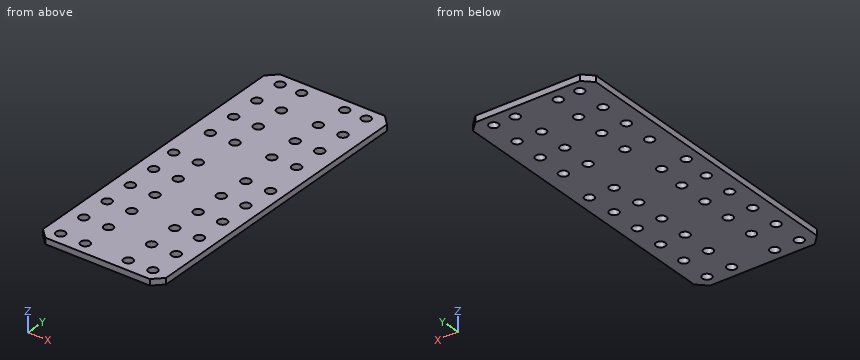
Autodesk Inventor part; units mm, degrees
ref_plane "YZ Plane" through (0, 0, 0) normal (1, 0, 0) x (0, 1, 0)
ref_plane "XZ Plane" through (0, 0, 0) normal (0, 1, 0) x (-1, 0, 0)
ref_plane "XY Plane" through (0, 0, 0) normal (0, 0, 1) x (1, 0, 0)
sketch "Sketch1" plane through (0, 0, 0) normal (0, 0, 1) x (1, 0, 0)
  circle A0 centre (-11, -99.1166) radius 1.5
  circle A1 centre (-13, -89.1166) radius 1.5
  circle A2 centre (-5, -89.1166) radius 1.5
  line L0 (0, -100.499) -> (0, -85.1166)
  line L1 (0, -85.1166) -> (-20, -85.1166)
  line L2 (-20, -85.1166) -> (-20, -111.0877)
  line L3 (-20, -111.0877) -> (-11.9783, -111.0877)
  line L4 (-11.9783, -111.0877) -> (-7.95, -105.7166)
  arc A3 (0, -100.499) -> (-7.95, -105.7166) centre (3.25, -114.1166) ccw
  circle A4 centre (-29, -99.1166) radius 1.5
  circle A5 centre (-27, -89.1166) radius 1.5
  circle A6 centre (-35, -89.1166) radius 1.5
  line L5 (-40, -100.499) -> (-40, -85.1166)
  arc A7 (-32.05, -105.7166) -> (-40, -100.499) centre (-43.25, -114.1166) ccw
  line L6 (-28.0217, -111.0877) -> (-32.05, -105.7166)
  line L7 (-20, -111.0877) -> (-28.0217, -111.0877)
  line L8 (-20, -85.1166) -> (-20, -111.0877)
  line L9 (-40, -85.1166) -> (-20, -85.1166)
  circle A8 centre (-6, 4) radius 1.5
  circle A9 centre (-10, 13) radius 1.5
  circle A10 centre (-13, 4) radius 1.5
  line L10 (-10, 23) -> (-10, 40)
  line L11 (-20, 40) -> (-10, 40)
  line L12 (-20, 0) -> (-20, 40)
  line L13 (0, 0) -> (-20, 0)
  line L14 (0, 0) -> (0, 8)
  line L15 (0, 8) -> (-10, 23)
  circle A11 centre (-34, 4) radius 1.5
  circle A12 centre (-30, 13) radius 1.5
  circle A13 centre (-27, 4) radius 1.5
  line L16 (-30, 23) -> (-30, 40)
  line L17 (-40, 8) -> (-30, 23)
  line L18 (-40, 0) -> (-40, 8)
  line L19 (-40, 0) -> (-20, 0)
  line L20 (-20, 0) -> (-20, 40)
  line L21 (-20, 40) -> (-30, 40)
  line L22 (0, 0) -> (-40, 0)
  line L23 (-40, 0) -> (-40, 8)
  line L24 (-40, 8) -> (0, 8)
  line L25 (0, 8) -> (0, 0)
  line L26 (0, -85.1166) -> (-40, -85.1166)
  line L27 (-40, -85.1166) -> (-40, -93.1166)
  line L28 (-40, -93.1166) -> (0, -93.1166)
  line L29 (0, -93.1166) -> (0, -85.1166)
  line L30 (0, -85.1166) -> (-40, -85.1166)
  line L31 (-40, -85.1166) -> (-40, 0)
  line L32 (-40, 0) -> (0, 0)
  line L33 (0, 0) -> (0, -85.1166)
  point P0 (0, -93.1166)
  dimension "d0" = 40
  dimension "d1" = 8
  dimension "d2" = 40
  dimension "d3" = 8
extrude "Extrusion1" add sketch "Sketch1" along normal blind 2 contours L28 L2 L1 L0 | L1 L9 L31 L19 L13 L33 | L28 L5 L9 L2 | L13 L12 L24 L14 | L19 L18 L24 L12
sketch "Sketch2" plane through (0, 0, 0) normal (0, 0, -1) x (-1, 0, 0)
  circle A0 centre (12.2614, -39.5) radius 1.5
  circle A1 centre (4.2614, -39.5) radius 1.5
  point P0 (0, 0)
extrude "Extrusion2" cut sketch "Sketch2" against normal blind 10
ref_plane "Work Plane1" through (-20, -93.1166, 0) normal (1, 0, 0) x (0, 0, -1)
mirror "Mirror1" about plane through (-20, -93.1166, 0) normal (1, 0, 0) of "Extrusion2"
sketch "Sketch3" plane through (0, 0, 0) normal (0, 0, -1) x (-1, 0, 0)
  circle A0 centre (35.7386, -39.5) radius 1.5
  circle A1 centre (27.7386, -39.5) radius 1.5
  circle A2 centre (4.2614, -39.5) radius 1.5
  circle A3 centre (12.2614, -39.5) radius 1.5
  line L0 (40, 8) -> (40, -93.1166)
  line L1 (0, 8) -> (40, 8)
  line L2 (0, -93.1166) -> (0, 8)
  line L3 (40, -93.1166) -> (0, -93.1166)
  circle A4 centre (13, 4) radius 1.5
  circle A5 centre (6, 4) radius 1.5
  circle A6 centre (27, 4) radius 1.5
  circle A7 centre (34, 4) radius 1.5
  circle A8 centre (35, -89.1166) radius 1.5
  circle A9 centre (27, -89.1166) radius 1.5
  circle A10 centre (5, -89.1166) radius 1.5
  circle A11 centre (13, -89.1166) radius 1.5
  circle A12 centre (6, 4) radius 1.5
  line L4 (6, 4) -> (6, -6)
  line L5 (6, -6) -> (6, -16)
  line L6 (6, -16) -> (6, -26)
  circle A13 centre (6, -6) radius 1.5
  circle A14 centre (6, -16) radius 1.5
  circle A15 centre (6, -26) radius 1.5
  circle A16 centre (5, -89.1166) radius 1.5
  line L7 (5, -89.1166) -> (5, -79.1166)
  line L8 (5, -79.1166) -> (5, -69.1166)
  line L9 (5, -69.1166) -> (5, -59.1166)
  line L10 (5, -59.1166) -> (5, -49.1166)
  circle A17 centre (5, -49.1166) radius 1.5
  circle A18 centre (5, -59.1166) radius 1.5
  circle A19 centre (5, -69.1166) radius 1.5
  circle A20 centre (5, -79.1166) radius 1.5
  circle A21 centre (14, -6) radius 1.5
  circle A22 centre (14, -16) radius 1.5
  circle A23 centre (14, -26) radius 1.5
  circle A24 centre (13, -49.1166) radius 1.5
  circle A25 centre (13, -59.1166) radius 1.5
  circle A26 centre (13, -69.1166) radius 1.5
  circle A27 centre (13, -79.1166) radius 1.5
  point P0 (0, 0)
  dimension "d8" = 10
  dimension "d9" = 10
  dimension "d10" = 10
  dimension "d11" = 3
  dimension "d12" = 3
  dimension "d13" = 3
  dimension "d14" = 10
  dimension "d15" = 10
  dimension "d16" = 10
  dimension "d17" = 10
  dimension "d18" = 3
  dimension "d19" = 3
  dimension "d20" = 3
  dimension "d21" = 3
  dimension "d24" = 8
extrude "Extrusion3" cut sketch "Sketch3" against normal blind 10 contours A15 | A14 L6 L5 | L5 L6 A14 | A13 L5 L4 | L4 L5 A13 | A17 | A18 L10 L9 | L9 L10 A18 | A19 L9 L8 | L8 L9 A19 | A20 L8 L7 | L7 L8 A20 | A21 | A22 | A23 | A24 | A25 | A26 | A27
mirror "Mirror2" about plane through (-20, -93.1166, 0) normal (1, 0, 0) of "Extrusion3"
chamfer "Chamfer1" distance 3 angle 45 4 edges at (0, 8, 1) (0, -93.1166, 1) (-40, -93.1166, 1) (-40, 8, 1)
properties part number "body_bone_1"
Geometry: final body of the model. Coordinates: model frame, mm. Round coordinates to 2 decimals unless told otherwise and drop trailing zeros. Order: outer loops, then holes, each group sorted by start corner. A loop starts at its lowest first (then second) coordinate and runs counter-clockwise, first axis right, second up. Notation, with made-up numbers: (35.5, 76) - (55.5, 76) arc R27 cw to (55.5, 99) - close; hole circle Ø2 at (38.5, 76.25). An arc over 180 degrees is marked (long way). Write item = value, one per line. Start each with the question number.
Q1. Cut plane B-B on z = 1. Give the number of separate pieces and of enclosed holes in the cut face, and give its area (3 significant figures).
Q2. Pin query (flat end, axial travel): pin 1 (2.5 mm diameter, centred on x = -35, y = -49.12, fed in from +Z). Return the tip coordinate at first contact, or that it passes through.
Q3. Ray query, line 1 (Y direction, x = -37.5, z = 0.35); line 2 (Y direction, x = -2, z = 1.25). Return the intervals inside material, ascending. Write a range as from..to.
Q4. Cut plane A-A on y = -26. Return the cut outline in (x, z), and give its area (3 significant figures).
Outcome:
q1.separate_pieces = 1
q1.enclosed_holes = 40
q1.area = 3,740 mm^2
q2.pin_1 = through
q3.line_1 = -92.62..7.5
q3.line_2 = -92.12..7
q4.outline = (-40, 0) - (-35.5, 0) - (-35.5, 2) - (-40, 2) - close; (-32.5, 0) - (-27.5, 0) - (-27.5, 2) - (-32.5, 2) - close; (-24.5, 0) - (-15.5, 0) - (-15.5, 2) - (-24.5, 2) - close; (-12.5, 0) - (-7.5, 0) - (-7.5, 2) - (-12.5, 2) - close; (-4.5, 0) - (0, 0) - (0, 2) - (-4.5, 2) - close
q4.area = 56.0 mm^2
